Answer from the drawing. Dimensions are ordinates in mm from the lowest x, y and z of the part. Round coordinates to 2 decimals unless told otherwise and drop trailing zeros. Loops run counter-clockwise (first coordinate to the right, second up) from the corner with the lowest first, then second, coordinate; pieces in that order, holes last. Notation, with made-up numbers: M 59.25,0.25 L 112.25,0.25 A17 cw 112.25,30.25 Z; hole C 23,45 d11. An arc over 180 degrees is marked long. Write each question's results on one line, items separated by ' | '.
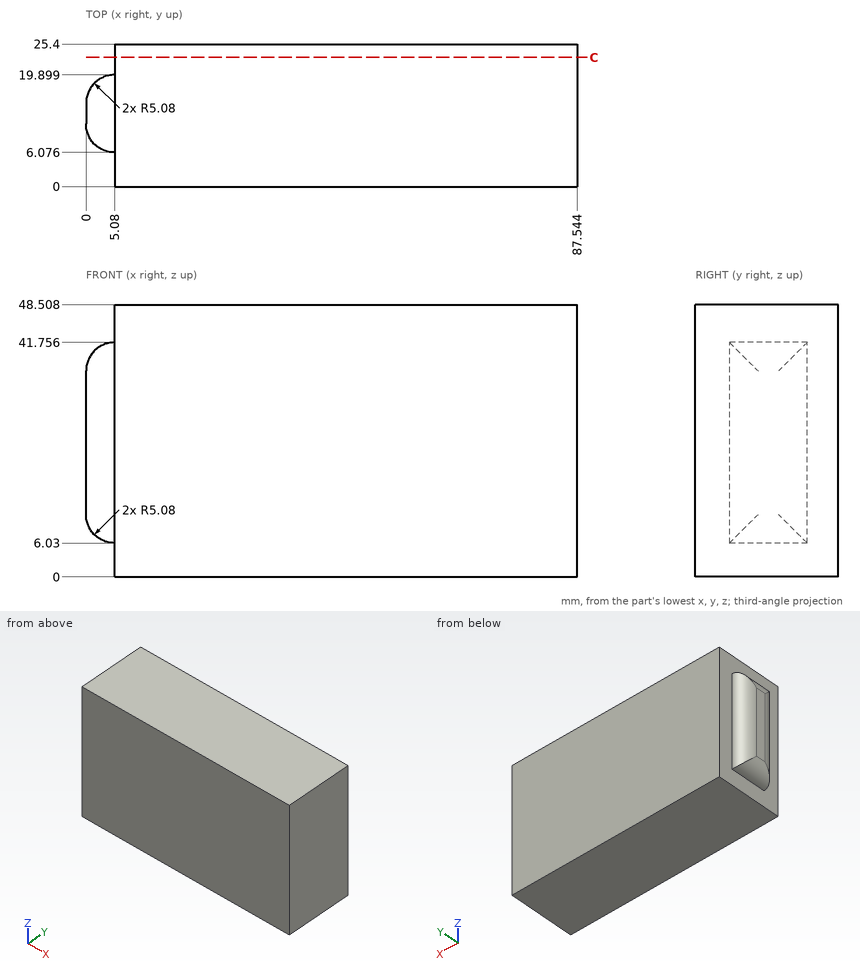
1. Find the intervals of material crossed by L1, parallel to X at y = 2, z = 28; L2, parallel to X at y = 7.25, z = 37 (1 decimal), in increasing order.
Completed:
L1: x = 5.08 to 87.54 | L2: x = 1.8 to 87.5
2. Given P1, Ø12, axis at y = 5, z = 11, coming from the -X side, flat-ended and moving along its own axis, determine where the tip first touches the part or whether it passes through.
Completed:
P1: stops at x = 0
3. Find section C-C, the plane y = 23. Give the vertices of the cut face in (x, z), then the cut area to 3 significant figures.
Completed:
outline: M 5.08,0 L 87.54,0 L 87.54,48.51 L 5.08,48.51 Z | area: 4,000 mm2
